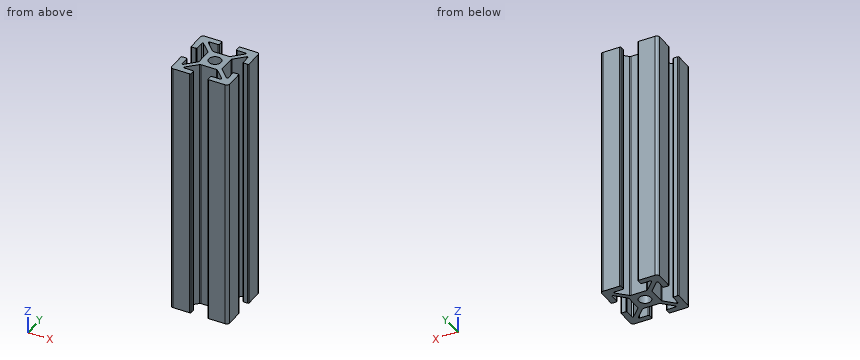
Autodesk Inventor part; units mm, degrees
ref_plane "YZ Plane" through (0, 0, 0) normal (1, 0, 0) x (0, 1, 0)
ref_plane "XZ Plane" through (0, 0, 0) normal (0, 1, 0) x (-1, 0, 0)
ref_plane "XY Plane" through (0, 0, 0) normal (0, 0, 1) x (1, 0, 0)
sketch "Skizze1" plane through (0, 0, 0) normal (0, 0, 1) x (1, 0, 0)
  line L0 (-20.0059, 0) -> (20.0059, 0)
  line L1 (0, -20.0059) -> (0, 20.0059)
  line L2 (-14.2899, 0) -> (14.2899, 0)
  line L3 (0, -14.2899) -> (0, 14.2899)
  line L4 (-10, -10) -> (10, 10) construction
  line L5 (10, -10) -> (-10, 10) construction
  line L6 (-8, -8) -> (8, 8) construction
  line L7 (8, -8) -> (-8, 8) construction
  line L8 (-2.7322, -4) -> (2.7322, -4)
  line L9 (4, -2.7322) -> (4, 2.7322)
  line L10 (2.7322, 4) -> (-2.7322, 4)
  line L11 (-4, 2.7322) -> (-4, -2.7322)
  line L12 (-4, -4) -> (4, 4) construction
  line L13 (4, -4) -> (-4, 4) construction
  arc A0 (-9, 10) -> (-10, 9) centre (-9, 9) ccw
  arc A1 (10, 9) -> (9, 10) centre (9, 9) ccw
  arc A2 (9, -10) -> (10, -9) centre (9, -9) ccw
  arc A3 (-10, -9) -> (-9, -10) centre (-9, -9) ccw
  line L14 (-3, 9.7) -> (-3, 8.3)
  line L15 (3, 9.7) -> (3, 8.3)
  line L16 (6.2151, 8) -> (3.3, 8)
  line L17 (-3.3, 8) -> (-6.2151, 8)
  line L18 (9, 10) -> (3.3, 10)
  line L19 (-3.3, 10) -> (-9, 10)
  line L20 (-9.7, -3) -> (-8.3, -3)
  line L21 (-9.7, 3) -> (-8.3, 3)
  line L22 (-8, 6.2151) -> (-8, 3.3)
  line L23 (-8, -3.3) -> (-8, -6.2151)
  line L24 (-10, 9) -> (-10, 3.3)
  line L25 (-10, -3.3) -> (-10, -9)
  line L26 (-3, -8.3) -> (-3, -9.7)
  line L27 (3, -8.3) -> (3, -9.7)
  line L28 (-9, -10) -> (-3.3, -10)
  line L29 (3.3, -10) -> (9, -10)
  line L30 (-6.2151, -8) -> (-3.3, -8)
  line L31 (3.3, -8) -> (6.2151, -8)
  line L32 (8.3, 3) -> (9.7, 3)
  line L33 (8.3, -3) -> (9.7, -3)
  line L34 (8, -6.2151) -> (8, -3.3)
  line L35 (8, 3.3) -> (8, 6.2151)
  line L36 (10, -9) -> (10, -3.3)
  line L37 (10, 3.3) -> (10, 9)
  arc A4 (-10, 3.3) -> (-9.7, 3) centre (-9.7, 3.3) ccw
  arc A5 (-8.3, 3) -> (-8, 3.3) centre (-8.3, 3.3) ccw
  arc A6 (-9.7, -3) -> (-10, -3.3) centre (-9.7, -3.3) ccw
  arc A7 (-8, -3.3) -> (-8.3, -3) centre (-8.3, -3.3) ccw
  arc A8 (-3.3, -10) -> (-3, -9.7) centre (-3.3, -9.7) ccw
  arc A9 (-3, -8.3) -> (-3.3, -8) centre (-3.3, -8.3) ccw
  arc A10 (3, -9.7) -> (3.3, -10) centre (3.3, -9.7) ccw
  arc A11 (3.3, -8) -> (3, -8.3) centre (3.3, -8.3) ccw
  arc A12 (8.3, -3) -> (8, -3.3) centre (8.3, -3.3) ccw
  arc A13 (10, -3.3) -> (9.7, -3) centre (9.7, -3.3) ccw
  arc A14 (8, 3.3) -> (8.3, 3) centre (8.3, 3.3) ccw
  arc A15 (9.7, 3) -> (10, 3.3) centre (9.7, 3.3) ccw
  arc A16 (3, 8.3) -> (3.3, 8) centre (3.3, 8.3) ccw
  arc A17 (3.3, 10) -> (3, 9.7) centre (3.3, 9.7) ccw
  arc A18 (-3.3, 8) -> (-3, 8.3) centre (-3.3, 8.3) ccw
  arc A19 (-3, 9.7) -> (-3.3, 10) centre (-3.3, 9.7) ccw
  line L38 (-7.4879, 6.4272) -> (-4.1464, 3.0858)
  line L39 (-6.4272, 7.4879) -> (-3.0858, 4.1464)
  line L40 (-6.4272, -7.4879) -> (-3.0858, -4.1464)
  line L41 (-7.4879, -6.4272) -> (-4.1464, -3.0858)
  arc A20 (-7.4879, 6.4272) -> (-8, 6.2151) centre (-7.7, 6.2151) ccw
  arc A21 (-6.2151, 8) -> (-6.4272, 7.4879) centre (-6.2151, 7.7) ccw
  arc A22 (-8, -6.2151) -> (-7.4879, -6.4272) centre (-7.7, -6.2151) ccw
  arc A23 (-6.4272, -7.4879) -> (-6.2151, -8) centre (-6.2151, -7.7) ccw
  line L42 (6.4272, -7.4879) -> (3.0858, -4.1464)
  line L43 (4.1464, -3.0858) -> (7.4879, -6.4272)
  arc A24 (6.2151, -8) -> (6.4272, -7.4879) centre (6.2151, -7.7) ccw
  arc A25 (7.4879, -6.4272) -> (8, -6.2151) centre (7.7, -6.2151) ccw
  line L44 (4.1464, 3.0858) -> (7.4879, 6.4272)
  line L45 (3.0858, 4.1464) -> (6.4272, 7.4879)
  arc A26 (6.4272, 7.4879) -> (6.2151, 8) centre (6.2151, 7.7) ccw
  arc A27 (8, 6.2151) -> (7.4879, 6.4272) centre (7.7, 6.2151) ccw
  arc A28 (-3.0858, 4.1464) -> (-2.7322, 4) centre (-2.7322, 4.5) ccw
  arc A29 (-4, 2.7322) -> (-4.1464, 3.0858) centre (-4.5, 2.7322) ccw
  arc A30 (2.7322, 4) -> (3.0858, 4.1464) centre (2.7322, 4.5) ccw
  arc A31 (4.1464, 3.0858) -> (4, 2.7322) centre (4.5, 2.7322) ccw
  arc A32 (-4.1464, -3.0858) -> (-4, -2.7322) centre (-4.5, -2.7322) ccw
  arc A33 (-2.7322, -4) -> (-3.0858, -4.1464) centre (-2.7322, -4.5) ccw
  arc A34 (3.0858, -4.1464) -> (2.7322, -4) centre (2.7322, -4.5) ccw
  arc A35 (4, -2.7322) -> (4.1464, -3.0858) centre (4.5, -2.7322) ccw
  circle A36 centre (0, 0) radius 2.1
  point P0 (3, 8.9014)
  point P1 (-3, 9.1415)
  point P2 (-8.9764, -3)
  point P3 (-9.1265, 3)
  point P4 (3, -9.1251)
  point P5 (-3, -9.1251)
  point P6 (9.1101, -3)
  point P7 (9.1101, 3)
  dimension "d0" = 20
  dimension "d1" = 20
  dimension "d2" = 16
  dimension "d3" = 16
  dimension "d4" = 8
  dimension "d5" = 8
  dimension "d6" = 1
  dimension "d7" = 6
  dimension "d8" = 6
  dimension "d9" = 6
  dimension "d10" = 6
  dimension "d11" = 0.3
  dimension "d12" = 1.5
  dimension "d13" = 1.5
  dimension "d14" = 0.3
  dimension "d15" = 1.5
  dimension "d16" = 0.3
  dimension "d17" = 1.5
  dimension "d18" = 0.3
  dimension "d19" = 0.5
  dimension "d20" = 4.2
  dimension "d21" = 45
  dimension "d22" = 10
  dimension "d23" = 10
  dimension "d24" = 4
  dimension "d25" = 4
  dimension "d26" = 10
  dimension "d27" = 8
  dimension "d28" = 4
  dimension "d29" = 4
  dimension "d30" = 10
  dimension "d31" = 9.1101
  dimension "d32" = 8
  dimension "d33" = 4
  dimension "d34" = 8.9014
  dimension "d35" = 9.1251
  dimension "d36" = 9.1415
  dimension "d37" = 8.9764
  dimension "d38" = 9.1265
extrude "Extrusion1" add sketch "Skizze1" against normal blind 88
sketch "Skizze2" plane through (0, 0, 0) normal (0, 0, 1) x (1, 0, 0)
  arc A0 (-4.1464, -3.0858) -> (-4, -2.7322) centre (-4.5, -2.7322) ccw
  line L0 (-4.1464, -3.0858) -> (-7.4879, -6.4272)
  arc A1 (-8, -6.2151) -> (-7.4879, -6.4272) centre (-7.7, -6.2151) ccw
  line L1 (-8, -6.2151) -> (-8, -3.3)
  arc A2 (-8, -3.3) -> (-8.3, -3) centre (-8.3, -3.3) ccw
  line L2 (-8.3, -3) -> (-9.7, -3)
  arc A3 (-9.7, -3) -> (-10, -3.3) centre (-9.7, -3.3) ccw
  line L3 (-10, -3.3) -> (-10, -9)
  arc A4 (-10, -9) -> (-9, -10) centre (-9, -9) ccw
  line L4 (-9, -10) -> (-3.3, -10)
  arc A5 (-3.3, -10) -> (-3, -9.7) centre (-3.3, -9.7) ccw
  line L5 (-3, -9.7) -> (-3, -8.3)
  arc A6 (-3, -8.3) -> (-3.3, -8) centre (-3.3, -8.3) ccw
  line L6 (-3.3, -8) -> (-6.2151, -8)
  arc A7 (-6.4272, -7.4879) -> (-6.2151, -8) centre (-6.2151, -7.7) ccw
  line L7 (-6.4272, -7.4879) -> (-3.0858, -4.1464)
  arc A8 (-2.7322, -4) -> (-3.0858, -4.1464) centre (-2.7322, -4.5) ccw
  line L8 (-2.7322, -4) -> (2.7322, -4)
  arc A9 (3.0858, -4.1464) -> (2.7322, -4) centre (2.7322, -4.5) ccw
  line L9 (3.0858, -4.1464) -> (6.4272, -7.4879)
  arc A10 (6.2151, -8) -> (6.4272, -7.4879) centre (6.2151, -7.7) ccw
  line L10 (6.2151, -8) -> (3.3, -8)
  arc A11 (3.3, -8) -> (3, -8.3) centre (3.3, -8.3) ccw
  line L11 (3, -8.3) -> (3, -9.7)
  arc A12 (3, -9.7) -> (3.3, -10) centre (3.3, -9.7) ccw
  line L12 (3.3, -10) -> (9, -10)
  arc A13 (9, -10) -> (10, -9) centre (9, -9) ccw
  line L13 (10, -9) -> (10, -3.3)
  arc A14 (10, -3.3) -> (9.7, -3) centre (9.7, -3.3) ccw
  line L14 (9.7, -3) -> (8.3, -3)
  arc A15 (8.3, -3) -> (8, -3.3) centre (8.3, -3.3) ccw
  line L15 (8, -3.3) -> (8, -6.2151)
  arc A16 (7.4879, -6.4272) -> (8, -6.2151) centre (7.7, -6.2151) ccw
  line L16 (7.4879, -6.4272) -> (4.1464, -3.0858)
  arc A17 (4, -2.7322) -> (4.1464, -3.0858) centre (4.5, -2.7322) ccw
  line L17 (4, -2.7322) -> (4, 2.7322)
  arc A18 (4.1464, 3.0858) -> (4, 2.7322) centre (4.5, 2.7322) ccw
  line L18 (4.1464, 3.0858) -> (7.4879, 6.4272)
  arc A19 (8, 6.2151) -> (7.4879, 6.4272) centre (7.7, 6.2151) ccw
  line L19 (8, 6.2151) -> (8, 3.3)
  arc A20 (8, 3.3) -> (8.3, 3) centre (8.3, 3.3) ccw
  line L20 (8.3, 3) -> (9.7, 3)
  arc A21 (9.7, 3) -> (10, 3.3) centre (9.7, 3.3) ccw
  line L21 (10, 3.3) -> (10, 9)
  arc A22 (10, 9) -> (9, 10) centre (9, 9) ccw
  line L22 (9, 10) -> (3.3, 10)
  arc A23 (3.3, 10) -> (3, 9.7) centre (3.3, 9.7) ccw
  line L23 (3, 9.7) -> (3, 8.3)
  arc A24 (3, 8.3) -> (3.3, 8) centre (3.3, 8.3) ccw
  line L24 (3.3, 8) -> (6.2151, 8)
  arc A25 (6.4272, 7.4879) -> (6.2151, 8) centre (6.2151, 7.7) ccw
  line L25 (6.4272, 7.4879) -> (3.0858, 4.1464)
  arc A26 (2.7322, 4) -> (3.0858, 4.1464) centre (2.7322, 4.5) ccw
  line L26 (2.7322, 4) -> (-2.7322, 4)
  arc A27 (-3.0858, 4.1464) -> (-2.7322, 4) centre (-2.7322, 4.5) ccw
  line L27 (-3.0858, 4.1464) -> (-6.4272, 7.4879)
  arc A28 (-6.2151, 8) -> (-6.4272, 7.4879) centre (-6.2151, 7.7) ccw
  line L28 (-6.2151, 8) -> (-3.3, 8)
  arc A29 (-3.3, 8) -> (-3, 8.3) centre (-3.3, 8.3) ccw
  line L29 (-3, 8.3) -> (-3, 9.7)
  arc A30 (-3, 9.7) -> (-3.3, 10) centre (-3.3, 9.7) ccw
  line L30 (-3.3, 10) -> (-9, 10)
  arc A31 (-9, 10) -> (-10, 9) centre (-9, 9) ccw
  line L31 (-10, 9) -> (-10, 3.3)
  arc A32 (-10, 3.3) -> (-9.7, 3) centre (-9.7, 3.3) ccw
  line L32 (-9.7, 3) -> (-8.3, 3)
  arc A33 (-8.3, 3) -> (-8, 3.3) centre (-8.3, 3.3) ccw
  line L33 (-8, 3.3) -> (-8, 6.2151)
  arc A34 (-7.4879, 6.4272) -> (-8, 6.2151) centre (-7.7, 6.2151) ccw
  line L34 (-7.4879, 6.4272) -> (-4.1464, 3.0858)
  arc A35 (-4, 2.7322) -> (-4.1464, 3.0858) centre (-4.5, 2.7322) ccw
  line L35 (-4, 2.7322) -> (-4, -2.7322)
  line L36 (-14.2899, 0) -> (14.2899, 0)
  line L37 (0, -14.2899) -> (0, 14.2899)
  circle A36 centre (0, 0) radius 2.1
  dimension "d41" = 4.2
extrude "Extrusion2" cut sketch "Skizze2" against normal blind 88 contours A36 L37 L36 | L36 L37 A36 | L37 A36 L36 | L36 A36 L37
properties part number "I Strebe waagrecht kurz" material "Aluminium 6061"
Build history of the part. All positions in model axes, mm. Give positions to 0.01 mm unless a question says otherwise; leave off trailing zeros. Loops run counter-clockwise (first coordinate to the right, second up) from the corner with the lowest first, then second, coordinate; pieces in that order, holes last. Notation, with made-up numbers: (-24, 65) - (-6, 65) arc R11 ccw to (-6, 80) - close; hole circle Ø10 at (86.25, 86). An arc over 180 degrees is marked (long way). Write item = value, one per line. Start each with the question number.
1) Probe probe 1 along Y at (x, z) = (0, -54.5); probe 2 along X at (y, z) = (6, -51). List the from-to ranges inside material, lowest first. Write a range as from..to.
2) Drop a flat-ended pin along its axis: pin 1 Ø2 at (x, z) = (-1.5, -37) entering from +Y. Give the stop position or say it passes through.
3) Band-saw the part on A-A on x = 0. Give the cut face in (y, z).
Final values:
q1.probe_1 = -4..-2.1, 2.1..4
q1.probe_2 = -10..-8, -7.06..-4.94, 4.94..7.06, 8..10
q2.pin_1 = 4
q3.outline = (-4, -88) - (-2.1, -88) - (-2.1, 0) - (-4, 0) - close; (2.1, -88) - (4, -88) - (4, 0) - (2.1, 0) - close
